Could you check a few things on this model? Use its own coordinates, in mm. A direction names the side the tool comes from. Round coordinates to 2 decimals unless told otherwise and drop trailing zeros. Loops run counter-clockwise (first coordinate to the right, second up) from the corner with the lowest first, then second, coordinate; pieces in that order, holes last. Notation, with made-up numbers: (-14, 47.5) -> (38, 47.5) arc R31 ccw to (38, 76.5) -> close; hole circle Ø1 at (71.5, 75). An arc over 180 degrees is marked (long way). One line per item, written item: value.
Solid Edge part; units mm, degrees
sketch "Sketch1" plane through (0, 0, 0) normal (0, 0, 1) x (1, 0, 0)
  line L0 (-150, -100) -> (150, -100)
  line L1 (150, -100) -> (150, 100)
  line L2 (150, 100) -> (-150, 100)
  line L3 (-150, 100) -> (-150, -100)
  dimension "D1" = 150
  dimension "D2" = 150
extrude "Protrusion1" add sketch "Sketch1" along normal blind 5
sketch "Sketch2" plane through (0, 0, 0) normal (0, 0, -1) x (1, 0, 0)
  circle A0 centre (-130, 80) radius 10
  circle A1 centre (130, 80) radius 10
  circle A2 centre (130, -80) radius 10
  circle A3 centre (-130, -80) radius 10
  dimension "D1" = 130
  dimension "D2" = 130
extrude "ExtrudedProtrusion_2" add sketch "Sketch2" along normal blind 30
sketch "Sketch3" plane through (0, 0, 5) normal (0, 0, 1) x (1, 0, 0)
  line L0 (-150, -100) -> (150, -100)
  line L1 (150, -100) -> (150, 100)
  line L2 (150, 100) -> (-150, 100)
  line L3 (-150, 100) -> (-150, -100)
  line L4 (145, 95) -> (-145, 95)
  line L5 (-145, 95) -> (-145, -95)
  line L6 (-145, -95) -> (145, -95)
  line L7 (145, -95) -> (145, 95)
extrude "ExtrudedProtrusion_3" add sketch "Sketch3" along normal blind 25
sketch "Sketch4" plane through (0, 0, 30) normal (0, 0, 1) x (1, 0, 0)
  line L0 (-145, 80) -> (-145, -80)
  line L1 (145, -80) -> (-145, -80)
  line L2 (145, 80) -> (145, -80)
  line L3 (-145, 80) -> (145, 80)
  line L4 (-150, -100) -> (150, -100)
  line L5 (150, -100) -> (150, 100)
  line L6 (150, 100) -> (-150, 100)
  line L7 (-150, 100) -> (-150, -100)
extrude "ExtrudedProtrusion_5" add sketch "Sketch4" against normal blind 5
hole "Hole_1" at (140, 90, 30) direction (0, 0, -1) diameter 8 end up to next thread major 10 thread length 5
hole "Hole1" at (-140, -90, 30) direction (0, 0, -1) diameter 8 end up to next thread major 10 thread length 5
hole "Hole2" at (-140, 90, 30) direction (0, 0, -1) diameter 8 end up to next thread major 10 thread length 5
hole "Hole3" at (140, -90, 30) direction (0, 0, -1) diameter 8 end up to next thread major 10 thread length 5
(1) If I drill on L1, parallel to Y at x = -140, z = 26.1; L2, parallel to X at y = -90, z = 26; L3, parallel to X at y = -51, z = 27, over which ranges is the centre line in solid material (lowest first)?
Recorded:
L1: -100 to -94, -86 to -80, 80 to 86, 94 to 100
L2: -150 to -144, -136 to 136, 144 to 150
L3: -150 to -145, 145 to 150
(2) Thinking about a two-plate mould opening in Z: for faces 4 (the face through (2, 95, 15)), 5 (the face through (130, 80, -30)), 6 (the face through (-2, -87, 25)), 7 (the face through (-131.302, 89.915, -14.79)), which applies, released by +Z, released by -Z, zero draft, split by the parting line, or undercut?
Recorded:
face 4: undercut
face 5: released by -Z
face 6: undercut
face 7: zero draft
(3) If we section it at B-B, the plane y = -51: Please give me the cut outline in (x, z), then the cut area to 3 significant figures.
Recorded:
outline: (-150, 0) -> (150, 0) -> (150, 30) -> (145, 30) -> (145, 5) -> (-145, 5) -> (-145, 30) -> (-150, 30) -> close
area: 1,750 mm²
(4) I'm going to push flat-ended pins straight in: pin 1 Ø2 at (x, y) = (-9, 36.5) entering from +Z; pin 2 Ø16.5 at (x, y) = (-64.5, -87) entering from -Z; pin 3 Ø5 at (y, z) = (-72.5, -3) entering from -X. Where does each tip first touch, or does it pass through?
Recorded:
pin 1: z = 5
pin 2: z = 0
pin 3: x = -138.66
(5) If we section it at D-D, the plane x = -130: Please give me the cut outline in (y, z).
Recorded:
outline: (-100, 0) -> (-90, 0) -> (-90, -30) -> (-70, -30) -> (-70, 0) -> (70, 0) -> (70, -30) -> (90, -30) -> (90, 0) -> (100, 0) -> (100, 30) -> (80, 30) -> (80, 25) -> (95, 25) -> (95, 5) -> (-95, 5) -> (-95, 25) -> (-80, 25) -> (-80, 30) -> (-100, 30) -> close
(6) If we section it at A-A, the plane x = -99.5: Please give me the cut outline in (y, z), then the cut area to 3 significant figures.
Recorded:
outline: (-100, 0) -> (100, 0) -> (100, 30) -> (80, 30) -> (80, 25) -> (95, 25) -> (95, 5) -> (-95, 5) -> (-95, 25) -> (-80, 25) -> (-80, 30) -> (-100, 30) -> close
area: 1,400 mm²
(7) For faces 1 (the face through (-140, -80, -15)), 2 (the face through (-136.034, -89.479, 27.535)), 3 (the face through (-2, 88, 25)), which set-ups out of +Z, -Z, +X, -X, +Y, -Y let a thin tool reach every point of the face, with its end or its side?
Recorded:
face 1: -Z
face 2: +Z
face 3: none
(8) If we section it at C-C, the plane z = -22.5: Please give me the cut outline in (x, y).
Recorded:
outline: circle Ø20 at (-130, -80); circle Ø20 at (-130, 80); circle Ø20 at (130, -80); circle Ø20 at (130, 80)
